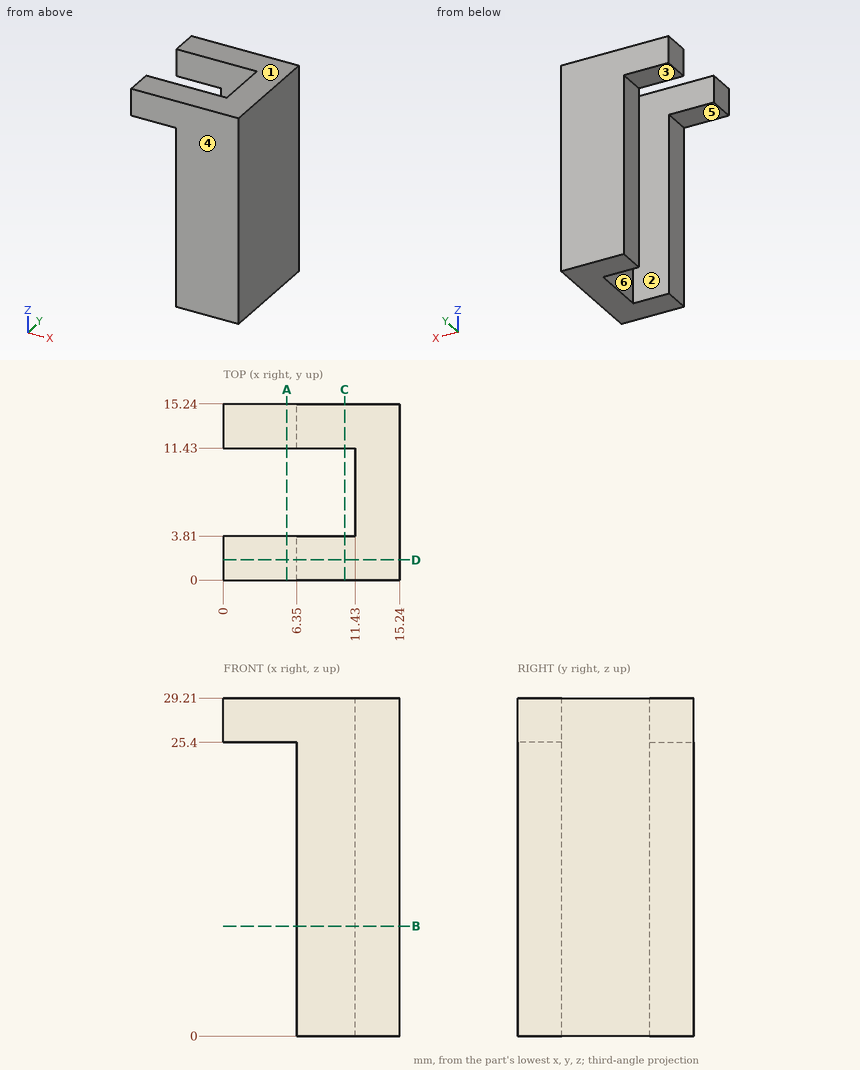
The figure shows three views and two pictorial views of one solid part (mm, origin at its lowest corner). Answer the questions. A direction names the side the tool comes from. Coordinates: 2 decimals unless noted, no trailing zeros. Order: outer loops, then holes, each group sorted by start corner. A loop starts at its lowest first (then second) coordinate and runs counter-clockwise, first axis right, second up.
Q1. For a pull along Y with two mould halves and no side action, classify the marked faces 4, 5 and 6 as pulls with the +Y half, pulls with the -Y half, needs draft (parallel to the pull), parting line crosses it, or undercut.
Q2. A cutting plane is placed at C-C, the plane x = 10.5. Write down the section's boundary in (y, z), and give its area (3 significant figures).
Q3. Which of the six approach directions +Z, -Z, +X, -X, +Y, -Y give full straight-line access (tool end or side, diameter ignored) to the marked faces 1, 2 and 3?
Q4. A cutting plane is placed at A-A, the plane x = 5.5. Write down the section's boundary in (y, z), and give its area (3 significant figures).
Q5. A cutting plane is placed at B-B, the plane z = 9.5. Write down the section's boundary in (x, y), and give its area (3 significant figures).
Q6. A cutting plane is placed at D-D, the plane y = 1.75. Write down the section's boundary in (x, z).
Q7. Given P1, Ø2, axis at y = 12, z = 14.5, coming from the -X side; P2, Ø4, axis at x = 1.5, y = 14, coming from the -Z side; P3, Ø2.5, axis at y = 6.5, z = 9.5, coming from the -X side; P4, Ø8, axis at x = 7, z = 9.5, coming from the -Y side, each flat-ended and moving along its own axis, determine where each tip first touches the part or whether it passes through.
Q8. Consider line 1 (Y direction, x = 7.25, z = 20); line 2 (X direction, y = 3.25, z = 23.75); line 3 (X direction, y = 10.25, z = 10.75). Determine where each line is inside the solid, lowest interval first.
Answers follow:
1. face 4: pulls with the -Y half
1. face 5: needs draft
1. face 6: undercut
2. outline: (0, 0) - (3.81, 0) - (3.81, 29.21) - (0, 29.21) - close; (11.43, 0) - (15.24, 0) - (15.24, 29.21) - (11.43, 29.21) - close
2. area: 223 mm2
3. face 1: +Z, +X, -X, +Y, -Y
3. face 2: +Z, -Z, -X
3. face 3: -Z, -X, +Y, -Y
4. outline: (0, 25.4) - (3.81, 25.4) - (3.81, 29.21) - (0, 29.21) - close; (11.43, 25.4) - (15.24, 25.4) - (15.24, 29.21) - (11.43, 29.21) - close
4. area: 29.0 mm2
5. outline: (6.35, 0) - (15.24, 0) - (15.24, 15.24) - (6.35, 15.24) - (6.35, 11.43) - (11.43, 11.43) - (11.43, 3.81) - (6.35, 3.81) - close
5. area: 96.8 mm2
6. outline: (0, 25.4) - (6.35, 25.4) - (6.35, 0) - (15.24, 0) - (15.24, 29.21) - (0, 29.21) - close
7. P1: stops at x = 6.35
7. P2: stops at z = 25.4
7. P3: stops at x = 11.43
7. P4: stops at y = 0
8. line 1: y = 0 to 3.81, 11.43 to 15.24
8. line 2: x = 6.35 to 15.24
8. line 3: x = 11.43 to 15.24
